Geometry check sheet. Reference: drawing and pictorial views, mm from the part's lowest x, y, z. Coordinates: 2 decimals unless noted, no trailing zeros. Loops run counter-clockwise (first coordinate to the right, second up) from the corner with the lowest first, then second, coordinate; pieces in that order, holes last. Notation, with made-up numbers: (16, 6.5) - (20, 6.5) arc R32 ccw to (20, 38.5) - close; hole circle Ø9 at (40, 38.5). An arc over 180 degrees is marked (long way). Use a Markdown table: item, result. Add a question column.
1) Go/stop test with flat-tipped pins: P1, Ø1, axis at y = 38, z = 2.5, coming from the +X side; P2, Ø3.5, axis at x = 44.45, y = 17.46, coming from the -Z side; P3, Ø1.6, axis at x = 4, z = 2.5, coming from the +Y side (1 decimal); P4, Ø1, axis at y = 52, z = 2, coming from the -X side. Record where each tip stops, or that it passes through.
2) Sectioned sample at B-B, the plane y = 7.5. Enter the section's corners in (x, z) (1 decimal).
3) Thickness scan on line 1 (Y direction, x = 44.45, z = 1.9) (1 decimal); line 2 (X direction, y = 9.5, z = 2.7) (1 decimal); line 3 (X direction, y = 35, z = 0.85). Record the ranges inside material, lowest first.
4) Sectioned sample at C-C, the plane z = 0.6. State how many separate pieces and enclosed holes the cut face has, then the cut area to 3 significant figures.
5) Sectioned sample at D-D, the plane x = 28.5. Enter the section's corners in (y, z) (1 decimal), then the cut area to 3 significant figures.
6) Sectioned sample at A-A, the plane x = 44.45. Enter the section's corners in (y, z) (1 decimal).
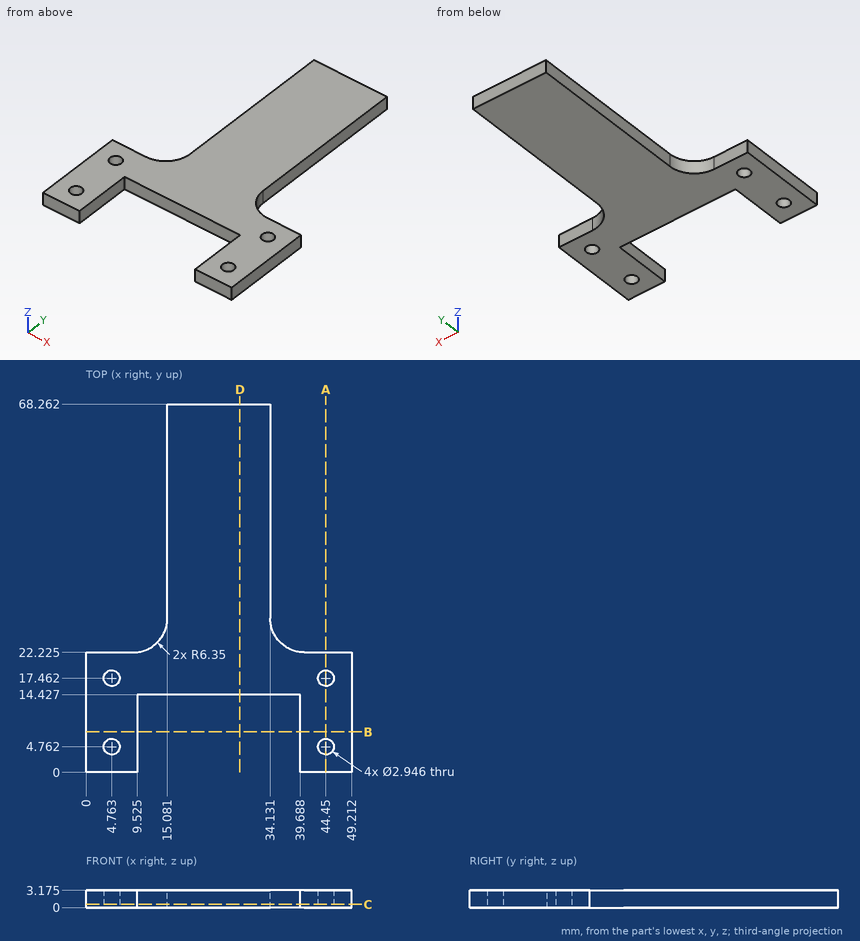
Solved:
| question | item | result |
|---|---|---|
| 1 | P1 | stops at x = 34.13 |
| 1 | P2 | stops at z = 0 |
| 1 | P3 | stops at y = 22.2 |
| 1 | P4 | stops at x = 15.08 |
| 2 | outline | (0, 0) - (9.5, 0) - (9.5, 3.2) - (0, 3.2) - close; (39.7, 0) - (49.2, 0) - (49.2, 3.2) - (39.7, 3.2) - close |
| 3 | line 1 | y = 0 to 3.3, 6.2 to 16, 18.9 to 22.2 |
| 3 | line 2 | x = 0 to 9.5, 39.7 to 49.2 |
| 3 | line 3 | x = 15.08 to 34.13 |
| 4 | separate pieces | 1 |
| 4 | enclosed holes | 4 |
| 4 | area | 1,530 mm2 |
| 5 | outline | (14.4, 0) - (68.3, 0) - (68.3, 3.2) - (14.4, 3.2) - close |
| 5 | area | 171 mm2 |
| 6 | outline | (0, 0) - (3.3, 0) - (3.3, 3.2) - (0, 3.2) - close; (6.2, 0) - (16, 0) - (16, 3.2) - (6.2, 3.2) - close; (18.9, 0) - (22.2, 0) - (22.2, 3.2) - (18.9, 3.2) - close |
